from build123d import *

# Parameters (mm, degrees)
F0_R     = 8.907425
F1_DEPTH = 30
F2_DEPTH = 30


with BuildPart() as f1:
    # F0 (on Front) → F1 (new body)
    with BuildSketch(Plane.XZ):
        with BuildLine():
            ThreePointArc((4.778965, -24.538979), (19.293446, -15.89852), (25, 0))
            ThreePointArc((25, 0), (19.452619, 15.703364), (5.27235, 24.437723))
            ThreePointArc((5.27235, 24.437723), (-24.998732, 0.251834), (4.778965, -24.538979))
        make_face()
        with BuildLine():
            ThreePointArc((5.27235, 11.345945), (10.547302, 6.729233), (12.511121, 0))
            ThreePointArc((12.511121, 0), (10.547302, -6.729233), (5.27235, -11.345945))
            ThreePointArc((5.27235, -11.345945), (-12.511121, 0), (5.27235, 11.345945))
        make_face(mode=Mode.SUBTRACT)
        with BuildLine():
            ThreePointArc((5.27235, 24.437723), (19.452619, 15.703364), (25, 0))
            ThreePointArc((25, 0), (19.293446, -15.89852), (4.778965, -24.538979))
            Line((4.778965, -24.538979), (69.271411, -14.982295))
            ThreePointArc((69.271411, -14.982295), (55.068389, 1.430734), (72.129728, 14.848039))
            Line((72.129728, 14.848039), (5.27235, 24.437723))
        make_face()
        with BuildLine():
            ThreePointArc((85, 0), (81.334591, 9.824818), (72.129728, 14.848039))
            ThreePointArc((72.129728, 14.848039), (55.068389, 1.430734), (69.271411, -14.982295))
            ThreePointArc((69.271411, -14.982295), (80.3458, -10.861143), (85, 0))
        make_face()
        with Locations((70, 0)):
            Circle(F0_R, mode=Mode.SUBTRACT)
    extrude(amount=F1_DEPTH)

    # F0 (on Front) → F2 (join)
    with BuildSketch(Plane.XZ):
        with BuildLine():
            ThreePointArc((5.27235, -11.345945), (10.547302, -6.729233), (12.511121, 0))
            ThreePointArc((12.511121, 0), (10.547302, 6.729233), (5.27235, 11.345945))
            Line((5.27235, 11.345945), (5.27235, -11.345945))
        make_face()
    extrude(amount=F2_DEPTH)


solid = f1.part
Build history of the part. All positions in model axes, mm. A direction names the side the tool comes from. Coordinates: 2 decimals unless noted, no trailing zeros. Order: outer loops, then holes, each group sorted by start corner. A loop starts at its lowest first (then second) coordinate and runs counter-clockwise, first axis right, second up. Notation, with made-up numbers: (69, 6) -> (103, 6) arc R19 ccw to (103, 28) -> close; hole circle Ø4 at (58.25, -28.5). An arc over 180 degrees is marked (long way). One line per item, written item: value.
(1) Mould opens along Z. For faces 3 (the flat face through (39.169, -14.79, 19.576)), 4 (the flat face through (36.57, -14.79, -19.83)), 5 (the cylindrical face through (78.23, -14.79, -3.41)) say: pulls with the +Z half, pulls with the -Z half, needs draft (parallel to the pull), parting line crosses it, or undercut.
Checked values:
face 3: pulls with the +Z half
face 4: pulls with the -Z half
face 5: undercut
(2) Drop flat-ended pins along their axis: pin 1 Ø6 at (x, y) = (2.5, -23) entering from -Z; pin 2 Ø1.5 at (x, y) = (57.5, -17.5) entering from -Z; pin 3 Ø1.5 at (y, z) = (-17.5, -2) entering from +X. Give the stop position or say it passes through.
Checked values:
pin 1: z = -25
pin 2: z = -16.84
pin 3: x = 84.95
(3) Slice it at C-C, the plane z = -3. List the corners of the cut face in (x, y), plus the area to 3 significant figures.
Checked values:
outline: (-24.82, -30) -> (-12.15, -30) -> (-12.15, 0) -> (-24.82, 0) -> close; (5.27, -30) -> (61.61, -30) -> (61.61, 0) -> (5.27, 0) -> close; (78.39, -30) -> (84.7, -30) -> (84.7, 0) -> (78.39, 0) -> close
area: 2,260 mm2
(4) Probe line 1 (Z direction, x = 0, y = -21); line 2 (X direction, y = -2, z = 7); line 3 (Z direction, x = 69, y = -15.25). List the from-to ranges inside material, lowest first. Write a range as [from, to].
Checked values:
line 1: [-25, -12.51], [12.51, 25]
line 2: [-24, -10.37], [5.27, 64.49], [75.51, 83.27]
line 3: [-15.02, -8.85], [8.85, 15.3]
(5) Slice it at B-B, the plane y = -20.5. List the corners of the cut face in (x, z), plus the area to 3 significant figures.
Checked values:
outline: (4.78, -24.54) -> (69.27, -14.98) arc R15 ccw to (72.13, 14.85) -> (5.27, 24.44) arc R25 ccw (long way) to start; hole (5.27, -11.35) -> (5.27, 11.35) arc R12.51 ccw (long way) to start; hole circle Ø17.81 at (70, 0)
area: 3,530 mm2
(6) Tool access for faces 1 (the flat face through (5.272, -15, 0)), 2 (the flat face through (29, -30, 0)): list every direction of +Z, -Z, +X, -X, +Y, -Y with a clear straight run to the whole face (end or side of a thin tool).
Checked values:
face 1: +Y, -Y
face 2: +Z, -Z, +X, -X, -Y
(7) Slice it at D-D, the plane x = 74.5. List the corners of the cut face in (y, z), plus the area to 3 significant figures.
Checked values:
outline: (-30, -14.31) -> (0, -14.31) -> (0, -7.69) -> (-30, -7.69) -> close; (-30, 7.69) -> (0, 7.69) -> (0, 14.31) -> (-30, 14.31) -> close
area: 397 mm2
(8) Slice it at A-A, the plane x = 0. List the corners of the cut face in (y, z).
Checked values:
outline: (-30, -25) -> (0, -25) -> (0, -12.51) -> (-30, -12.51) -> close; (-30, 12.51) -> (0, 12.51) -> (0, 25) -> (-30, 25) -> close
